Geometry: see drawing. Coordinates: mm, zero at the bounding-box minimum. A direction names the side the tool comes from. Round coordinates to 2 decimals unless told otherwise and drop trailing zeros. Loops run counter-clockwise (first coordinate to the right, second up) from the corner with the lowest first, then second, coordinate; pieces in that order, holes last. Notation, with made-up numbers: (88, 87) -> (123, 87) arc R26 ccw to (123, 125) -> close; hole circle Ø6 at (45, 40). An arc over 180 degrees is marked (long way). Answer in a Markdown table with one row per item.
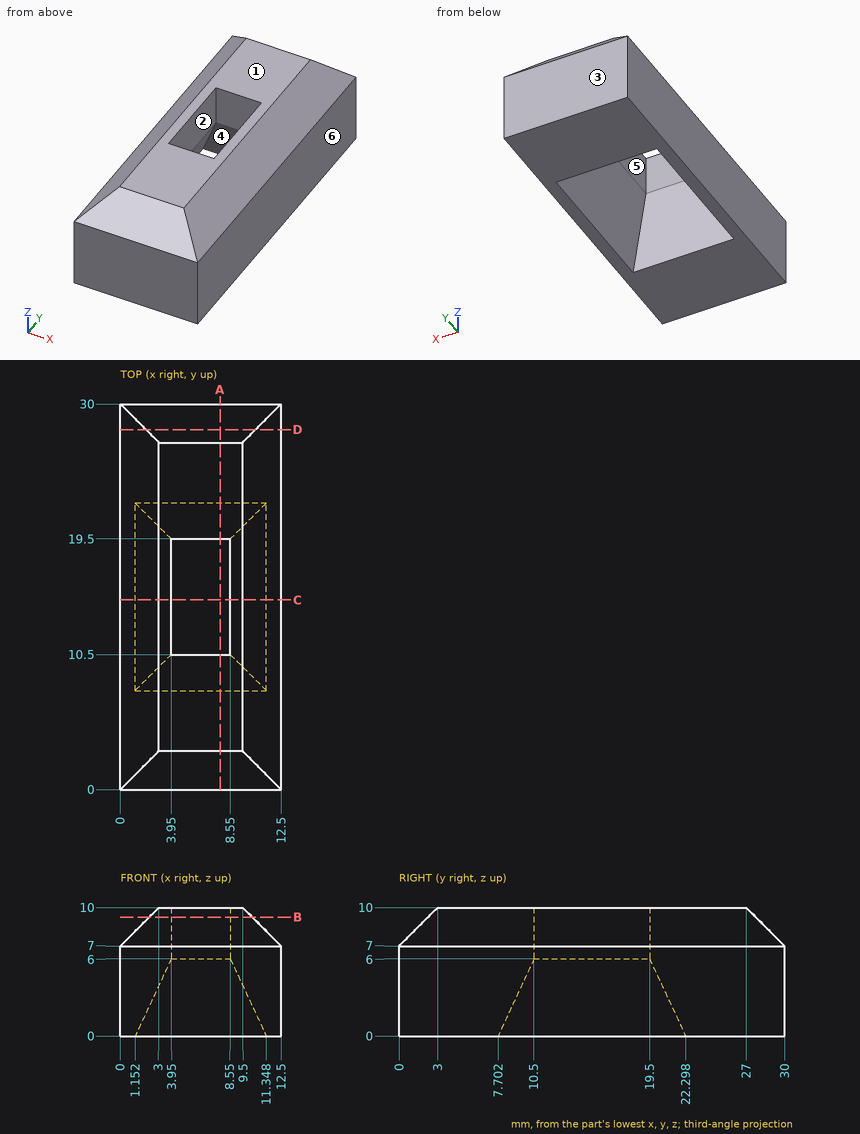
Item 1: Section query B-B, the plane z = 9.25. Output: boundary loops of the cut face in (x, y).
Ans:
| item | result |
|---|---|
| outline | (2.25, 2.25) -> (10.25, 2.25) -> (10.25, 27.75) -> (2.25, 27.75) -> close; hole (3.95, 10.5) -> (8.55, 10.5) -> (8.55, 19.5) -> (3.95, 19.5) -> close |
Item 2: Section query A-A, the plane x = 7.75. Output: boundary loops of the cut face in (y, z), and give its area (3 significant figures).
Ans:
| item | result |
|---|---|
| outline | (0, 0) -> (7.7, 0) -> (10.5, 6) -> (10.5, 10) -> (3, 10) -> (0, 7) -> close; (19.5, 6) -> (22.3, 0) -> (30, 0) -> (30, 7) -> (27, 10) -> (19.5, 10) -> close |
| area | 184 mm2 |
Item 3: Set-up query: the marked faces 4, 5 and 6. Return all of +Z, -Z, +X, -X, +Y, -Y with unobstructed straight access to the full face (end or side cutting, diameter ignored); none if empty.
Ans:
| item | result |
|---|---|
| face 4 | -Z |
| face 5 | +Z, -Z |
| face 6 | +Z, -Z, +X, +Y, -Y |
Item 4: Ray query, L1, parallel to Y at x = 4.25, z = 6.25; L2, parallel to X at y = 20.25, z = 3.5; L3, parallel to X at y = 12.25, z = 1.75. Return the intervals inside material, ascending.
Ans:
| item | result |
|---|---|
| L1 | 0 to 10.5, 19.5 to 30 |
| L2 | 0 to 2.78, 9.72 to 12.5 |
| L3 | 0 to 1.97, 10.53 to 12.5 |
Item 5: Mould query, pull axis Y, two halves, no side actions, for the marked faces 1, 2 and 3. Classes: released by +Y, released by -Y, zero draft, split by the parting line, or undercut.
Ans:
| item | result |
|---|---|
| face 1 | zero draft |
| face 2 | undercut |
| face 3 | released by +Y |
Item 6: Section query D-D, the plane y = 28. Output: boundary loops of the cut face in (x, z).
Ans:
| item | result |
|---|---|
| outline | (0, 0) -> (12.5, 0) -> (12.5, 7) -> (10.5, 9) -> (2, 9) -> (0, 7) -> close |
Item 7: First-contact query: P1, Ø1.2, axis at x = 7, z = 9, coming from the +Y side; P2, Ø1.5, axis at x = 6, z = 8.5, coming from the +Y side. Flat tips, straight axial feed; report the tip coordinate or a pass-through.
Ans:
| item | result |
|---|---|
| P1 | y = 28.6 |
| P2 | y = 29.25 |
Item 8: Section query C-C, the plane y = 14.75. Output: boundary loops of the cut face in (x, z).
Ans:
| item | result |
|---|---|
| outline | (0, 0) -> (1.15, 0) -> (3.95, 6) -> (3.95, 10) -> (3, 10) -> (0, 7) -> close; (8.55, 6) -> (11.35, 0) -> (12.5, 0) -> (12.5, 7) -> (9.5, 10) -> (8.55, 10) -> close |
